Input: dimensioned drawing with shaded views. Units: mm. Origin: part minimum x, y, z. A direction names the side the tool comes from. Round coordinates to 2 decimals unless told otherwise and drop trailing zeros. Order: outer loops, then holes, each group sorted by start corner. A loop starts at its lowest first (then second) coordinate and runs counter-clockwise, first axis right, second up. Notation, with made-up numbers: (80.25, 9) - (99.25, 9) arc R34 ccw to (99.25, 40) - close; hole circle Ø10 at (-21.5, 52). An arc over 180 degrees is marked (long way). Return JSON: item names as keys, results as strings. Group by question number.
1) Section D-D, the plane x = 24.25. Return loops of the section in (y, z).
2) Contact query for flat-ended pins moving along their axis: P1, Ø4, axis at x = 22, z = 1.5, coming from the -Y side; P2, Ø1.5, axis at x = 16, y = 18, coming from the -Z side; P3, Ø3, axis at y = 19.5, z = 3.5, coming from the +X side; P4, Ø1.5, axis at x = 20, z = 1, coming from the -Y side. Output: stop coordinate, or through.
3) Section C-C, the plane y = 6. Return loops of the section in (x, z).
4) Ray query, line 1 (Z direction, x = 18, y = 26.25); line 2 (Y direction, x = 12.25, z = 4.5); line 3 (Y direction, x = 8.5, z = 4). Return the intervals inside material, ascending. Write a range as from..to.
5) Section A-A, the plane x = 14. Return loops of the section in (y, z), plus the area to 3 significant figures.
6) Access query for the marked faces 1 and 2. Directions: +Z, -Z, +X, -X, +Y, -Y. A direction counts if a zero-diameter tool reaches every point of the face in a straight line with its end or side. Return the directions, or none.
7) Mould query, pull axis X, two halves, no side actions, for the marked faces 3, 4 and 5. Classes: pulls with the +X half, pulls with the -X half, needs draft (parallel to the pull), parting line crosses it, or undercut.
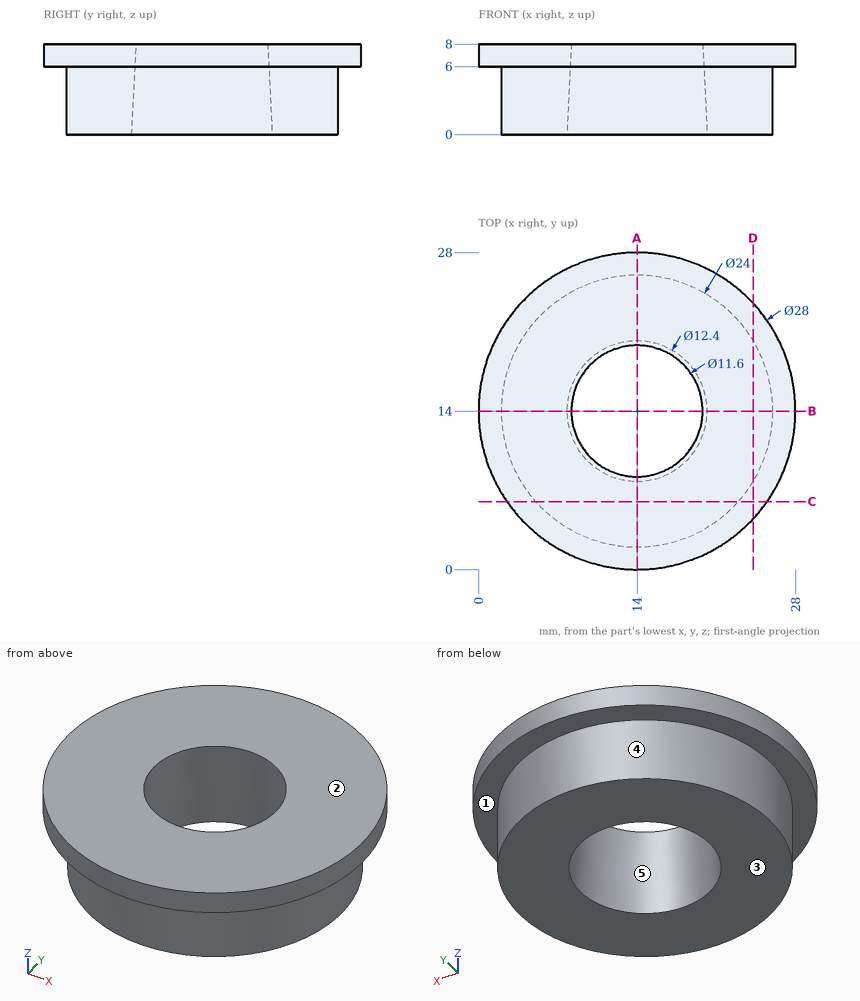
Geometry check:
{
 "1": {"outline": "(4.46, 6) - (7.76, 6) - (7.76, 0) - (20.24, 0) - (20.24, 6) - (23.54, 6) - (23.54, 8) - (4.46, 8) - close"},
 "2": {"P1": "y = 3.61", "P2": "through", "P3": "x = 25.31", "P4": "y = 3.21"},
 "3": {"outline": "(2.51, 6) - (5.06, 6) - (5.06, 0) - (22.94, 0) - (22.94, 6) - (25.49, 6) - (25.49, 8) - (2.51, 8) - close"},
 "4": {"line 1": "6..8", "line 2": "2.13..8.29, 19.71..25.87", "line 3": "3.33..11.6, 16.4..24.67"},
 "5": {"outline": "(0, 6) - (2, 6) - (2, 0) - (7.8, 0) - (8.2, 8) - (0, 8) - close; (19.8, 8) - (20.2, 0) - (26, 0) - (26, 6) - (28, 6) - (28, 8) - close", "area": "104 mm2"},
 "6": {"face 1": "-Z", "face 2": "+Z, +X, -X, +Y, -Y"},
 "7": {"face 3": "needs draft", "face 4": "parting line crosses it", "face 5": "undercut"}
}
